Answer from the drawing. Dimensions are ordinates in mm from the lowest x, y and z of the part. A direction names the side the tool comes from. Coordinates: 2 decimals unless noted, no trailing zeros. Loops run counter-clockwise (first coordinate to the right, second up) from the corner with the lowest first, then second, coordinate; pieces in that order, holes last. Notation, with made-up numbers: M -2.5,15.25 L 33.5,15.25 A19 ccw 33.5,20.25 Z; hole C 50,-4.75 d6. An arc over 180 degrees is marked long. One line per item, written item: value. Start each with the question number.
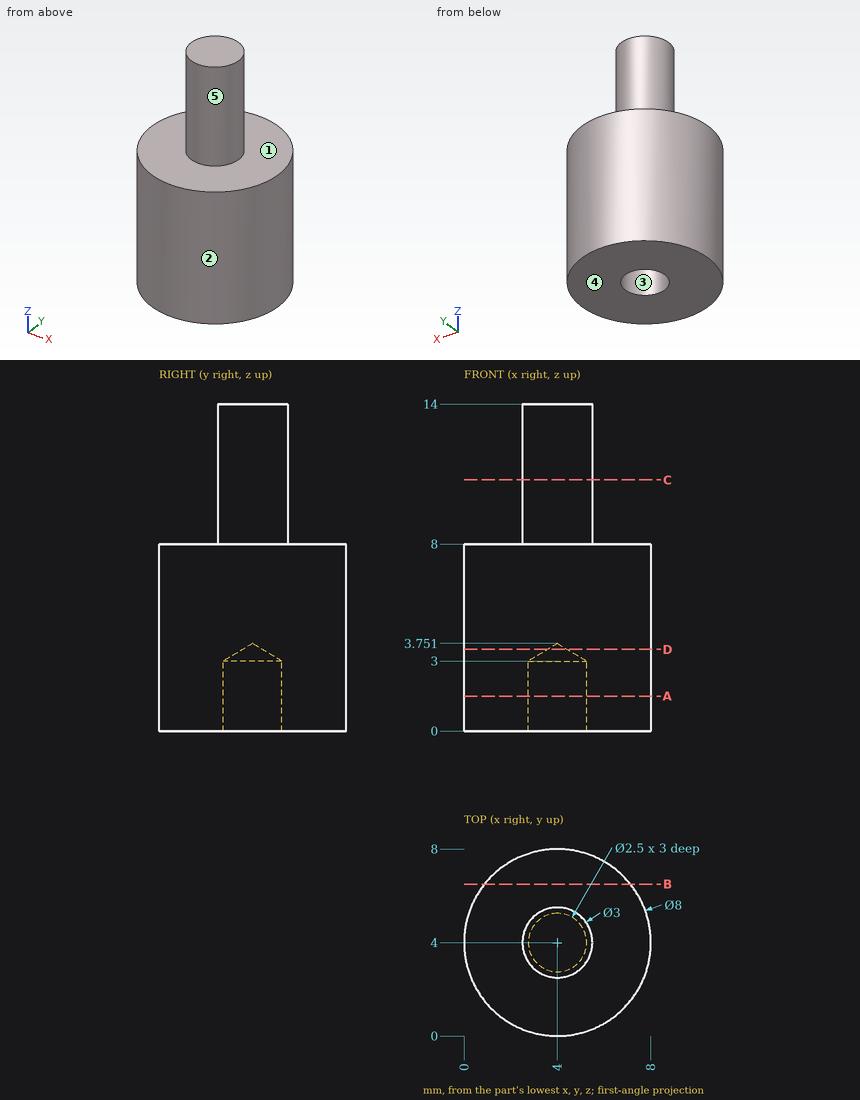
1) Flat-ended cylindrical pins translate along their axes: pin 1 (2 mm diameter, centred on y = 1, z = 10.5, fed in from -X); pin 2 (2.5 mm diameter, centred on x = 3, y = 2.5, fed in from +Z); pin 3 (1.5 mm diameter, centred on x = 4, y = 4, fed in from -Z); pin 4 (1 mm diameter, centred on y = 6, z = 2, fed in from +X). Find the tip coordinate at first contact, or state that the pin passes through.
2) Section C-C (z = 10.75) is taken. Determine the outline of the cut face in (x, y), then the cut area to 3 significant figures.
3) For a pull along X with two mould halves and no side action, classify the marked faces 1, 2 and 3 as released by +X, released by -X, zero draft, split by the parting line, or undercut.
4) Section A-A (z = 1.5) is taken. Determine the outline of the cut face in (x, y), then the cut area to 3 significant figures.
5) Section D-D (z = 3.5) is taken. Determine the outline of the cut face in (x, y).
6) Section B-B (y = 6.5) is taken. Determine the outline of the cut face in (x, z), then the cut area to 3 significant figures.
7) Consider line 1 along Y through (x, z) = (4, 1.1); line 2 along Z through (x, y) = (5.75, 7.25); line 3 along X through (y, z) = (5, 0.5). Determine where each line is inside the solid, lowest interval first.
8) A tool of negligible diameter and unlimited length cuts with its end or side. For the marked faces 4 and 5, from which of +Z, -Z, +X, -X, +Y, -Y can it reach the whole face along a straight path? Write none if from no direction.
Results found:
1. pin 1: passes through
1. pin 2: stops at z = 14
1. pin 3: stops at z = 3.3
1. pin 4: stops at x = 7.71
2. outline: C 4,4 d3
2. area: 7.07 mm²
3. face 1: zero draft
3. face 2: split by the parting line
3. face 3: undercut
4. outline: C 4,4 d8; hole C 4,4 d2.5
4. area: 45.4 mm²
5. outline: C 4,4 d8; hole C 4,4 d0.84
6. outline: M 0.88,0 L 7.12,0 L 7.12,8 L 0.88,8 Z
6. area: 50.0 mm²
7. line 1: y = 0 to 2.75, 5.25 to 8
7. line 2: z = 0 to 8
7. line 3: x = 0.13 to 3.25, 4.75 to 7.87
8. face 4: -Z, +X, -X, +Y, -Y
8. face 5: +Z
